Check sheet for the modelled part. Datum: model origin and axes. Units: mm. Face numbers are marked on the shaded views. Give positions to 0.01 mm unless a question says otherwise; leave off trailing zeros. Write each loop counter-clockwise with the first axis right and the second up, starting at its lowest first coordinate (ties: lowest second). Pieces come first, ordered by that corner, then holes. Notation, with made-up numbers: (3.25, 22) -> (35.25, 22) arc R16 ccw to (35.25, 35) -> close; hole circle Ø10 at (-34, -20). An arc over 180 degrees is marked (long way). Return JSON: item names as keys, results as strings.
from build123d import *

# Parameters (mm, degrees)
SKETCH1_R           = 2.5
BOSS_EXTRUDE1_DEPTH = 3
SKETCH2_R           = 1.5
CUT_EXTRUDE1_DEPTH  = 77.127156728
FILLET1_R           = 10


with BuildPart() as part:
    # Sketch1 → Boss-Extrude1 (new body)
    with BuildSketch(Plane.XY):
        with BuildLine():
            Line((0, -19), (30, -19))
            Line((30, -19), (64.201367261, 15.201367261))
            Line((64.201367261, 15.201367261), (58.615223689, 20.787510832))
            Line((58.615223689, 20.787510832), (44.190245353, 35.212489168))
            Line((44.190245353, 35.212489168), (38.604101782, 40.798632739))
            Line((38.604101782, 40.798632739), (16.805469042, 19))
            Line((16.805469042, 19), (0, 19))
            ThreePointArc((0, 19), (-19, 0), (0, -19))
        make_face()
        Circle(SKETCH1_R, mode=Mode.SUBTRACT)
    extrude(amount=BOSS_EXTRUDE1_DEPTH)

    # Sketch2 → Cut-Extrude1 (cut, through all)
    with BuildSketch(Plane.XY.offset(3)):
        with Locations((38.878105659, 35.574881393)):
            Circle(SKETCH2_R)
        with Locations((58.977615915, 15.475371138)):
            Circle(SKETCH2_R)
    extrude(amount=-CUT_EXTRUDE1_DEPTH, mode=Mode.SUBTRACT)

    # Fillet1
    fillet1_edges = [part.edges().sort_by_distance(p)[0] for p in [
        (16.805469042, 19, 1.5),
        (30, -19, 1.5),
    ]]
    fillet(fillet1_edges, radius=FILLET1_R)


solid = part.part
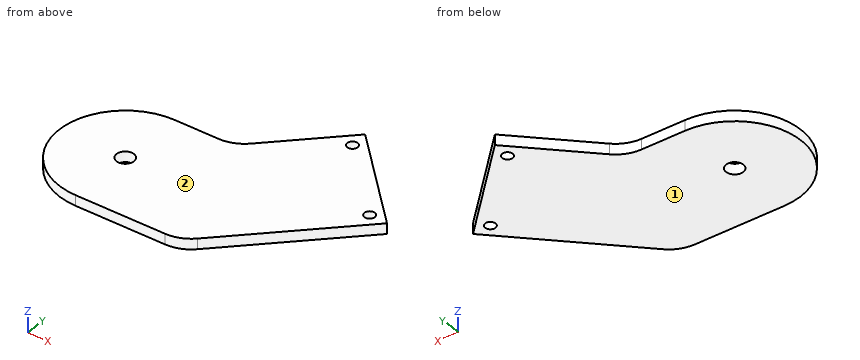
(1) Release check for a two-part mould opening along Z. For the marked faces 1 and 2 record: pulls with the +Z half, pulls with the -Z half, needs draft (parallel to the pull), parting line crosses it, or undercut.
Reply:
{"face 1": "pulls with the -Z half", "face 2": "pulls with the +Z half"}
(2) Cross-section at B-B on z = 0.7. Enter the section's corners in (x, y).
Reply:
{"outline": "(0, -19) -> (25.86, -19) arc R10 ccw to (32.93, -16.07) -> (64.2, 15.2) -> (38.6, 40.8) -> (19.73, 21.93) arc R10 cw to (12.66, 19) -> (0, 19) arc R19 ccw to start; hole circle Ø5 at (0, 0); hole circle Ø3 at (38.88, 35.57); hole circle Ø3 at (58.98, 15.48)"}
(3) Thickness scan on L1, parallel to X at y = 25.5, z = 0.7; L2, parallel to Y at x = 38.5, z = 1.7; L3, parallel to X at y = 7, z = 0.2. Record the ranges inside material, lowest first.
Reply:
{"L1": "23.31 to 53.9", "L2": "-10.5 to 34.12, 37.03 to 40.69", "L3": "-17.66 to 56"}
(4) Depth check by flat-ended pin: pin 1 Ø2 at (x, y) = (24, 26.5) entering from +Z; pin 2 Ø0.9 at (x, z) = (9, 1.5) entering from +Y; pin 3 Ø1.5 at (y, z) = (23.5, 0.5) entering from -X. Enter the tip coordinate at first touch or a pass-through.
Reply:
{"pin 1": "z = 3", "pin 2": "y = 19", "pin 3": "x = 20.56"}
(5) Cross-section at C-C on x = 4. Enter the section's corners in (y, z).
Reply:
{"outline": "(-19, 0) -> (19, 0) -> (19, 3) -> (-19, 3) -> close"}
(6) Cross-section at A-A on y = 0. Enter the section's corners in (x, z).
Reply:
{"outline": "(-19, 0) -> (-2.5, 0) -> (-2.5, 3) -> (-19, 3) -> close; (2.5, 0) -> (49, 0) -> (49, 3) -> (2.5, 3) -> close"}
(7) Cross-section at D-D on y = 6.5. Enter the section's corners in (x, z).
Reply:
{"outline": "(-17.85, 0) -> (55.5, 0) -> (55.5, 3) -> (-17.85, 3) -> close"}
